Verification items for the finished model (mm, model axes). A direction names the side the tool comes from. Give positions to 0.01 mm unless a question says otherwise; leave off trailing zeros. Order: outer loops, then holes, each group sorted by start corner. A loop starts at its lowest first (then second) coordinate and runs counter-clockwise, first axis right, second up. Notation, with made-up numbers: (64, -37) -> (94, -37) arc R27 ccw to (94, -6) -> close; hole circle Ø5 at (4, 86.5). An arc over 180 degrees is marked (long way). One line per question, with ' | ' between items. Start each with the question number.
Q1. Section check A-A on y = 18. Record the cut outline in (x, z), plus the area to 3 significant figures.
Q2. Section check C-C on y = 36.5. Record the cut outline in (x, z), plus the area to 3 significant figures.
Q3. Section check B-B on z = 1.25. Give the number of separate pieces and of enclosed holes in the cut face, plus the area to 3 significant figures.
Q4. Mould release check, pull along Y, two halves, no side actions. Record for faces 1 (the cylindrical face through (-5.246, -3.658, 1.972)), 2 (the cylindrical face through (-7.92, 9.59, 2.96)), 3 (the flat face through (3, 3, 4)), 4 (the flat face through (10, 33, 2)): released by +Y, released by -Y, zero draft, split by the parting line, or undercut.
Q5. Material ranges on probe 1 along Y at (x, z) = (-15.5, 0.5); probe 2 along Z at (x, y) = (-7, 1); probe 3 along Y at (x, z) = (-18.5, 1), recorded low to high. Write a range as [from, to].
Q6. Go/stop test with flat-tipped pins: pin 1 (4 mm diameter, centred on x = -3, y = 1, fed in from +Z); pin 2 (8 mm diameter, centred on x = 13, y = 36, fed in from -Z); pin 3 (6 mm diameter, centred on x = -33, y = 5, fed in from +Z). Record where each tip stops, or that it passes through.
Q7. Section check D-D on x = 0. Record the cut outline in (y, z), plus the area to 3 significant figures.
Q8. Access from +Z, -Z, +X, -X, +Y, -Y to the whole of each face (thin tool, end or side, straight path). Record for faces 5 (the flat face through (-3.257, 27.669, 2.958)), 6 (the cylindrical face through (9, 31, 1)).
from build123d import *

# Parameters (mm, degrees)
SKETCH1_R               = 3
SKETCH1_R_2             = 4
SKETCH1_R_3             = 2.5
BOSS_EXTRUDE1_DEPTH     = 6
CUT_EXTRUDE1_DEPTH      = 57.885850613
CUT_EXTRUDE1_DEPTH_BACK = 57.885850613
SKETCH4_R               = 7.5
CUT_EXTRUDE2_DEPTH      = 2
FILLET1_R               = 1
FILLET2_R               = 0.5
SKETCH5_R               = 5
CUT_EXTRUDE4_DEPTH      = 2


with BuildPart() as part:
    # Sketch1 → Boss-Extrude1 (new body)
    with BuildSketch(Plane.XY):
        with BuildLine():
            Line((16.72972973, 33.378378378), (6.535491145, 3.645182505))
            ThreePointArc((6.535491145, 3.645182505), (6.111138498, 1.921892634), (5.998106477, 0.150727223))
            ThreePointArc((5.998106477, 0.150727223), (2.637317184, -5.389300332), (-3.799375872, -4.643785415))
            ThreePointArc((-3.799375872, -4.643785415), (-5.267291655, -3.646275313), (-6.888425749, -2.923968315))
            Line((-6.888425749, -2.923968315), (-36.621621622, 7.27027027))
            ThreePointArc((-36.621621622, 7.27027027), (-39.99026822, 11.688193819), (-37.19776432, 16.49108361))
            Line((-37.19776432, 16.49108361), (9.80223568, 39.49108361))
            ThreePointArc((9.80223568, 39.49108361), (15.308172233, 38.749132763), (16.72972973, 33.378378378))
        make_face()
        with Locations((-35, 12)):
            Circle(SKETCH1_R, mode=Mode.SUBTRACT)
        Circle(SKETCH1_R_2, mode=Mode.SUBTRACT)
        with Locations((12, 35)):
            Circle(SKETCH1_R_3, mode=Mode.SUBTRACT)
    extrude(amount=BOSS_EXTRUDE1_DEPTH)

    # Sketch2 → Cut-Extrude1 (cut, two sides: drawn at the far end of the back side and taken through both)
    with BuildSketch(Plane.XY.offset(6).offset(-CUT_EXTRUDE1_DEPTH_BACK)):
        with BuildLine():
            Line((-24.859247394, 17.097563964), (-14.697085232, 22.070536937))
            ThreePointArc((-14.697085232, 22.070536937), (-13.551269449, 22.142130773), (-12.690430853, 21.38254115))
            Line((-12.690430853, 21.38254115), (-7.71745788, 11.220378988))
            ThreePointArc((-7.71745788, 11.220378988), (-7.940043134, 9.568598022), (-9.551269449, 9.142130773))
            Line((-9.551269449, 9.142130773), (-24.686404584, 14.331319962))
            ThreePointArc((-24.686404584, 14.331319962), (-25.696998564, 15.656697027), (-24.859247394, 17.097563964))
        make_face()
        with BuildLine():
            Line((-25.837837838, 10.972972973), (-10.702702703, 5.783783784))
            ThreePointArc((-10.702702703, 5.783783784), (-9.459459459, 3.243243243), (-12, 2))
            Line((-12, 2), (-27.135135135, 7.189189189))
            ThreePointArc((-27.135135135, 7.189189189), (-28.378378378, 9.72972973), (-25.837837838, 10.972972973))
        make_face()
        with BuildLine():
            Line((-9.097563964, 23.140752606), (-4.124590991, 12.978590444))
            ThreePointArc((-4.124590991, 12.978590444), (-2.683724054, 12.140839274), (-1.358346989, 13.151433254))
            Line((-1.358346989, 13.151433254), (3.8308422, 28.286568389))
            ThreePointArc((3.8308422, 28.286568389), (3.404374951, 29.897794704), (1.752593985, 30.120379958))
            Line((1.752593985, 30.120379958), (-8.409568177, 25.147406985))
            ThreePointArc((-8.409568177, 25.147406985), (-9.1691578, 24.286568389), (-9.097563964, 23.140752606))
        make_face()
        with BuildLine():
            Line((7.189189189, 27.135135135), (2, 12))
            ThreePointArc((2, 12), (3.243243243, 9.459459459), (5.783783784, 10.702702703))
            Line((5.783783784, 10.702702703), (10.972972973, 25.837837838))
            ThreePointArc((10.972972973, 25.837837838), (9.72972973, 28.378378378), (7.189189189, 27.135135135))
        make_face()
    extrude(amount=CUT_EXTRUDE1_DEPTH + CUT_EXTRUDE1_DEPTH_BACK, mode=Mode.SUBTRACT)

    # Sketch4 → Cut-Extrude2 (cut)
    with BuildSketch(Plane.XY.offset(6)):
        Circle(SKETCH4_R)
    extrude(amount=-CUT_EXTRUDE2_DEPTH, mode=Mode.SUBTRACT)

    # Fillet1
    fillet1_edges = [part.edges().sort_by_distance(p)[0] for p in [
        (6.54275782, 3.666376974, 5),
        (-6.909620217, -2.91670164, 5),
    ]]
    fillet(fillet1_edges, radius=FILLET1_R)

    # Fillet2
    # the kernel refuses this fillet: 0.5 mm, written as the material it adds along each edge
    with BuildSketch(Plane(origin=(0, 0, 4), x_dir=(0.7313195548489669, 0.6820349761526229, 0), z_dir=(0.6820349761526229, -0.7313195548489669, 0))) as fillet2_piece_1:
        with BuildLine():
            CenterArc((7.5 - FILLET2_R, FILLET2_R), FILLET2_R, 270, 90)
            Line((7.5 - FILLET2_R, 0), (7.5, 0))
            Line((7.5, 0), (7.5, FILLET2_R))
        make_face()
    revolve(axis=Axis((0, 0, 4), (0, 0, 1)), revolution_arc=146.144973872)
    with BuildSketch(Plane(origin=(6.216216216, 5.797297297, 4), x_dir=(0.6053689071166585, 0.7959450271823945, 0), z_dir=(-0.7959450271823945, 0.6053689071166585, 0))) as fillet2_piece_2_section:
        with BuildLine():
            CenterArc((1 + FILLET2_R, -FILLET2_R), FILLET2_R, 90, 90)
            Line((1, -FILLET2_R), (1, 0))
            Line((1, 0), (1 + FILLET2_R, 0))
        make_face()
    fillet2_piece_2 = revolve(axis=Axis((6.216216216, 5.797297297, 4), (0, 0, -1)), revolution_arc=189.741738526, mode=Mode.PRIVATE)
    fillet2_piece_2 = split(fillet2_piece_2, bisect_by=Plane(origin=(6.878990216, 4.647054795, 4.123474389), z_dir=(-0.945945945945946, 0.32432432432432406, 0)), keep=Keep.TOP, mode=Mode.PRIVATE)
    add(fillet2_piece_2)
    with BuildSketch(Plane(origin=(-8.391891892, -1.351351351, 4), x_dir=(0.9872813990461049, 0.1589825119236894, 0), z_dir=(-0.1589825119236894, 0.9872813990461049, 0))) as fillet2_piece_3_section:
        with BuildLine():
            CenterArc((1 + FILLET2_R, -FILLET2_R), FILLET2_R, 90, 90)
            Line((1 + FILLET2_R, 0), (1, 0))
            Line((1, 0), (1, -FILLET2_R))
        make_face()
    fillet2_piece_3 = revolve(axis=Axis((-8.391891892, -1.351351351, 4), (0, 0, -1)), revolution_arc=189.741738526, mode=Mode.PRIVATE)
    fillet2_piece_3 = split(fillet2_piece_3, bisect_by=Plane(origin=(-7.890298213, -2.580469184, 4.123474408), z_dir=(0.3243243243243243, 0.9459459459459462, 0)), keep=Keep.TOP, mode=Mode.PRIVATE)
    add(fillet2_piece_3)

    # Sketch5 → Cut-Extrude4 (cut)
    with BuildSketch(Plane(origin=(0, 0, 0), x_dir=(-1, 0, 0), z_dir=(0, 0, -1))):
        with Locations((-12, 35)):
            Circle(SKETCH5_R)
    extrude(amount=-CUT_EXTRUDE4_DEPTH, mode=Mode.SUBTRACT)


solid = part.part
Filled in:
1) outline: (-34.11, 0) -> (-23.02, 0) -> (-23.02, 6) -> (-34.11, 6) -> close; (-11.04, 0) -> (-6.58, 0) -> (-6.58, 6) -> (-11.04, 6) -> close; (0.3, 0) -> (4.06, 0) -> (4.06, 6) -> (0.3, 6) -> close; (8.29, 0) -> (11.46, 0) -> (11.46, 6) -> (8.29, 6) -> close | area: 135 mm²
2) outline: (3.69, 0) -> (7.23, 0) -> (7.23, 2) -> (10, 2) -> (10, 6) -> (3.69, 6) -> close; (14, 2) -> (16.77, 2) -> (16.77, 6) -> (14, 6) -> close | area: 43.4 mm²
3) separate pieces: 1 | enclosed holes: 6 | area: 840 mm²
4) face 1: released by -Y | face 2: undercut | face 3: zero draft | face 4: undercut
5) probe 1: [0.03, 3.2], [7.43, 11.18], [21.68, 27.11] | probe 2: [0, 4.01] | probe 3: [1.06, 4.23], [8.46, 12.21], [20.21, 25.64]
6) pin 1: z = 4 | pin 2: z = 2 | pin 3: z = 6
7) outline: (-6, 0) -> (-4, 0) -> (-4, 4) -> (-6, 4) -> close; (4, 0) -> (17.11, 0) -> (17.11, 6) -> (7.5, 6) -> (7.5, 4.5) arc R0.5 cw to (7, 4) -> (4, 4) -> close; (29.26, 0) -> (34.69, 0) -> (34.69, 6) -> (29.26, 6) -> close | area: 112 mm²
8) face 5: +Z, -Z | face 6: -Z
